from build123d import *

# Parameters (mm, degrees)
SALIENTE_EXTRUIR1_DEPTH = 81
CORTAR_EXTRUIR1_DEPTH   = 6
CROQUIS3_R              = 2
CORTAR_EXTRUIR2_DEPTH   = 81
CROQUIS4_R              = 4
CORTAR_EXTRUIR4_DEPTH   = 6
CORTAR_EXTRUIR5_DEPTH   = 71
CROQUIS7_R              = 2.75
CORTAR_EXTRUIR6_DEPTH   = 71
CORTAR_EXTRUIR7_DEPTH   = 6
CORTAR_EXTRUIR8_DEPTH   = 6
REDONDEO2_R             = 1
CROQUIS10_R             = 3
CORTAR_EXTRUIR9_DEPTH   = 71
CROQUIS15_W             = 12.5
CROQUIS15_H             = 20
CORTAR_EXTRUIR10_DEPTH  = 100


with BuildPart() as part:
    # Croquis1 → Saliente-Extruir1 (new body)
    with BuildSketch(Plane.XY):
        with BuildLine():
            Line((50, 0), (50, -150))
            Line((50, -150), (0, -150))
            Line((0, -150), (-50, -150))
            Line((-50, -150), (-50, 0))
            ThreePointArc((-50, 0), (0, 50), (50, 0))
        make_face()
        with BuildLine():
            Line((-35, 0), (-35, -77.5))
            ThreePointArc((-35, -77.5), (-32.071067812, -84.571067812), (-25, -87.5))
            Line((-25, -87.5), (25, -87.5))
            ThreePointArc((25, -87.5), (32.071067812, -84.571067812), (35, -77.5))
            Line((35, -77.5), (35, 0))
            ThreePointArc((35, 0), (0, 35), (-35, 0))
        make_face(mode=Mode.SUBTRACT)
    extrude(amount=SALIENTE_EXTRUIR1_DEPTH)

    # Croquis2 → Cortar-Extruir1 (cut)
    with BuildSketch(Plane(origin=(0, 0, 0), x_dir=(-1, 0, 0), z_dir=(0, 0, -1))):
        Polygon((4.907477288, 42.5), (2.453738644, 46.75), (-2.453738644, 46.75), (-4.907477288, 42.5), (-2.453738644, 38.25), (2.453738644, 38.25), align=None)
        Polygon((-42.5, 4.907477288), (-46.75, 2.453738644), (-46.75, -2.453738644), (-42.5, -4.907477288), (-38.25, -2.453738644), (-38.25, 2.453738644), align=None)
        Polygon((42.5, 4.907477288), (38.25, 2.453738644), (38.25, -2.453738644), (42.5, -4.907477288), (46.75, -2.453738644), (46.75, 2.453738644), align=None)
        Polygon((-42.5, -33.842522712), (-46.75, -36.296261356), (-46.75, -41.203738644), (-42.5, -43.657477288), (-38.25, -41.203738644), (-38.25, -36.296261356), align=None)
        Polygon((42.5, -33.842522712), (38.25, -36.296261356), (38.25, -41.203738644), (42.5, -43.657477288), (46.75, -41.203738644), (46.75, -36.296261356), align=None)
        Polygon((-42.5, -130.092522712), (-46.75, -132.546261356), (-46.75, -137.453738644), (-42.5, -139.907477288), (-38.25, -137.453738644), (-38.25, -132.546261356), align=None)
        Polygon((42.5, -139.907477288), (46.75, -137.453738644), (46.75, -132.546261356), (42.5, -130.092522712), (38.25, -132.546261356), (38.25, -137.453738644), align=None)
    extrude(amount=-CORTAR_EXTRUIR1_DEPTH, mode=Mode.SUBTRACT)

    # Croquis3 → Cortar-Extruir2 (cut)
    with BuildSketch(Plane.XY.offset(81)):
        with Locations((-15.5, -97.5)):
            Circle(CROQUIS3_R)
        with Locations((15.5, -97.5)):
            Circle(CROQUIS3_R)
        with Locations((15.5, -128.5)):
            Circle(CROQUIS3_R)
        with Locations((-15.5, -128.5)):
            Circle(CROQUIS3_R)
    extrude(amount=-CORTAR_EXTRUIR2_DEPTH, mode=Mode.SUBTRACT)

    # Croquis4 → Cortar-Extruir4 (cut)
    with BuildSketch(Plane(origin=(0, 0, 0), x_dir=(-1, 0, 0), z_dir=(0, 0, -1))):
        with Locations((-15.5, -97.5)):
            Circle(CROQUIS4_R)
        with Locations((15.5, -97.5)):
            Circle(CROQUIS4_R)
        with Locations((-15.5, -128.5)):
            Circle(CROQUIS4_R)
        with Locations((15.5, -128.5)):
            Circle(CROQUIS4_R)
    extrude(amount=-CORTAR_EXTRUIR4_DEPTH, mode=Mode.SUBTRACT)

    # Croquis6 → Cortar-Extruir5 (cut)
    with BuildSketch(Plane.XY.offset(81)):
        with BuildLine():
            Line((-30, -91), (30, -91))
            ThreePointArc((30, -91), (33.535533906, -92.464466094), (35, -96))
            Line((35, -96), (35, -130))
            ThreePointArc((35, -130), (33.535533906, -133.535533906), (30, -135))
            Line((30, -135), (-30, -135))
            ThreePointArc((-30, -135), (-33.535533906, -133.535533906), (-35, -130))
            Line((-35, -130), (-35, -96))
            ThreePointArc((-35, -96), (-33.535533906, -92.464466094), (-30, -91))
        make_face()
    extrude(amount=-CORTAR_EXTRUIR5_DEPTH, mode=Mode.SUBTRACT)

    # Croquis7 → Cortar-Extruir6 (cut)
    with BuildSketch(Plane.XY.offset(81)):
        with Locations((0, 40.605)):
            Circle(CROQUIS7_R)
        with Locations((28.71207085, 28.71207085)):
            Circle(CROQUIS7_R)
        with Locations((40.605, 0)):
            Circle(CROQUIS7_R)
        with Locations((28.71207085, -28.71207085)):
            Circle(CROQUIS7_R)
        with Locations((0, -40.605)):
            Circle(CROQUIS7_R)
        with Locations((-28.71207085, -28.71207085)):
            Circle(CROQUIS7_R)
        with Locations((-40.605, 0)):
            Circle(CROQUIS7_R)
        with Locations((-28.71207085, 28.71207085)):
            Circle(CROQUIS7_R)
    extrude(amount=-CORTAR_EXTRUIR6_DEPTH, mode=Mode.SUBTRACT)

    # Croquis8 → Cortar-Extruir7 (cut)
    with BuildSketch(Plane.XY.offset(81)):
        Polygon((4.907477288, 40.605), (2.453738644, 44.855), (-2.453738644, 44.855), (-4.907477288, 40.605), (-2.453738644, 36.355), (2.453738644, 36.355), align=None)
        Polygon((-23.987281715, 27.385533641), (-25.200861361, 32.140589664), (-29.925650495, 33.467126873), (-33.436859985, 30.038608059), (-32.223280339, 25.283552036), (-27.498491205, 23.957014828), align=None)
        Polygon((32.049942164, 25.114578887), (33.496525937, 29.804006221), (30.158654623, 33.401498184), (25.374199536, 32.309562813), (23.927615763, 27.62013548), (27.265487077, 24.022643516), align=None)
        Polygon((-40.605, -4.907477288), (-36.355, -2.453738644), (-36.355, 2.453738644), (-40.605, 4.907477288), (-44.855, 2.453738644), (-44.855, -2.453738644), align=None)
        Polygon((44.801667212, -2.543878465), (44.906396981, 2.362481184), (40.709729769, 4.906359649), (36.408332788, 2.543878465), (36.303603019, -2.362481184), (40.500270231, -4.906359649), align=None)
    extrude(amount=-CORTAR_EXTRUIR7_DEPTH, mode=Mode.SUBTRACT)

    # Croquis9 → Cortar-Extruir8 (cut)
    with BuildSketch(Plane(origin=(0, -87.5, 0), x_dir=(1, 0, 0), z_dir=(0, 1, 0))):
        with BuildLine():
            Line((-21, -120), (21, -120))
            Line((21, -120), (21, -47))
            ThreePointArc((21, -47), (19.535533906, -43.464466094), (16, -42))
            Line((16, -42), (-16, -42))
            ThreePointArc((-16, -42), (-19.535533906, -43.464466094), (-21, -47))
            Line((-21, -47), (-21, -120))
        make_face()
    extrude(amount=-CORTAR_EXTRUIR8_DEPTH, mode=Mode.SUBTRACT)

    # Redondeo2
    redondeo2_edges = [part.edges().sort_by_distance(p)[0] for p in [
        (21, -91, 64),
        (19.535533906, -91, 43.464466094),
        (0, -91, 42),
        (-19.535533906, -91, 43.464466094),
        (-21, -91, 64),
        (-21, -87.5, 64),
        (21, -87.5, 64),
        (19.535533906, -87.5, 43.464466094),
        (0, -87.5, 42),
        (-19.535533906, -87.5, 43.464466094),
    ]]
    fillet(redondeo2_edges, radius=REDONDEO2_R)

    # Croquis10 → Cortar-Extruir9 (cut)
    with BuildSketch(Plane(origin=(0, 0, 0), x_dir=(-1, 0, 0), z_dir=(0, 0, -1))):
        with Locations((0, 42.5)):
            Circle(CROQUIS10_R)
        with Locations((-42.5, 0)):
            Circle(CROQUIS10_R)
        with Locations((42.5, 0)):
            Circle(CROQUIS10_R)
        with Locations((42.5, -38.75)):
            Circle(CROQUIS10_R)
        with Locations((-42.5, -38.75)):
            Circle(CROQUIS10_R)
        with Locations((-42.5, -135)):
            Circle(CROQUIS10_R)
        with Locations((42.5, -135)):
            Circle(CROQUIS10_R)
    extrude(amount=-CORTAR_EXTRUIR9_DEPTH, mode=Mode.SUBTRACT)

    # Croquis15 → Cortar-Extruir10 (cut)
    with BuildSketch(Plane(origin=(50, 0, 0), x_dir=(0, 0, -1), z_dir=(1, 0, 0))):
        with Locations((-16.25, -112.839909006)):
            Rectangle(CROQUIS15_W, CROQUIS15_H)
    extrude(amount=-CORTAR_EXTRUIR10_DEPTH, mode=Mode.SUBTRACT)


solid = part.part
The listing builds one solid part. Answer for the finished solid, in the listing's coordinates (mm). A direction names the side the tool comes from. Coordinates: 2 decimals unless noted, no trailing zeros. Put each result on its own line as item: value.
1. Determine the mould class of faces 1 (the face through (0.77, 34.99, 39.93)), 2 (the face through (-50, -76, 40)), 3 (the face through (1, -150, 40)) for opening direction Y: pulls with the +Y half, pulls with the -Y half, needs draft (parallel to the pull), parting line crosses it, or undercut.
Answer sheet:
face 1: undercut
face 2: needs draft
face 3: pulls with the -Y half
2. The part is cut by section A-A on x = 0. State how many separate pieces and enclosed holes the cut face has, plus the area to 3 significant figures.
Answer sheet:
separate pieces: 3
enclosed holes: 0
area: 2,400 mm^2
3. A tool of negligible diameter and unlimited length cuts with its end or side. For faces 4 (the face through (38.6, -2.1, 75)), 5 (the face through (-42, -102.84, 16)), 6 (the face through (-17.2, -130.2, 6)), from which of +Z, -Z, +X, -X, +Y, -Y can it reach the whole face along a straight path? Write none if from no direction.
Answer sheet:
face 4: +Z
face 5: +X, -X
face 6: -Z
4. Flat-ended cylindrical pins translate along their axes: pin 1 Ø2.5 at (x, y) = (41.5, -133) entering from -Z; pin 2 Ø12 at (x, y) = (1.5, 26.5) entering from +Z; pin 3 Ø2.5 at (x, y) = (-2, 41.5) entering from +Z; pin 4 Ø3 at (x, z) = (29.5, 22) entering from +Y. Find the tip coordinate at first contact, or state that the pin passes through.
Answer sheet:
pin 1: stops at z = 6
pin 2: passes through
pin 3: stops at z = 75
pin 4: stops at y = 41.42
5. Find the intervals of material crossed by line 1 along X through (y, z) = (-128, 3); line 2 along Y through (x, z) = (15.5, 7.1); line 3 along Y through (x, z) = (-42, 40), in increasing order. Write a range as from..to.
Answer sheet:
line 1: x = -50..-19.47, -11.53..11.53, 19.47..50
line 2: y = -150..-130.5, -126.5..-99.5, -95.5..-87.5, 31.38..47.54
line 3: y = -150..-137.96, -132.04..-41.71, -35.79..-2.96, 2.96..27.13
